```python
from build123d import *

# Parameters (mm, degrees)
ESBO_O1_R                = 3.35
RESSALTO_EXTRUS_O1_DEPTH = 10
ESBO_O2_R                = 1.75
CORTE_EXTRUS_O1_DEPTH    = 10
ESBO_O3_W                = 10.1
ESBO_O3_H                = 5
CORTE_EXTRUS_O2_DEPTH    = 20


with BuildPart() as part:
    # Esboço1 → Ressalto-extrusão1 (new body)
    with BuildSketch(Plane.XY):
        Polygon((-8, -5), (-8, -15), (8, -15), (8, -5), (20, -5), (20, 0), (-20, 0), (-20, -5), align=None)
        with Locations((0, -6.75)):
            Circle(ESBO_O1_R, mode=Mode.SUBTRACT)
    extrude(amount=RESSALTO_EXTRUS_O1_DEPTH)

    # Esboço2 → Corte-extrusão1 (cut)
    with BuildSketch(Plane(origin=(0, 0, 0), x_dir=(1, 0, 0), z_dir=(0, 1, 0))):
        with Locations(Location((-15, -5, 0), (0, 0, 180))):
            Circle(ESBO_O2_R)
        with Locations(Location((15, -5, 0), (0, 0, 180))):
            Circle(ESBO_O2_R)
    extrude(amount=-CORTE_EXTRUS_O1_DEPTH, mode=Mode.SUBTRACT)

    # Esboço3 → Corte-extrusão2 (cut)
    with BuildSketch(Plane.XZ.offset(15)):
        with Locations((0, 5)):
            Rectangle(ESBO_O3_W, ESBO_O3_H)
    extrude(amount=-CORTE_EXTRUS_O2_DEPTH, mode=Mode.SUBTRACT)


solid = part.part
```
Read the model definition and answer for the solid it produces. Units are mm, in the model's axes. A direction names the side the tool comes from. Coordinates: 2 decimals unless noted, no trailing zeros. Write each loop counter-clockwise with the first axis right and the second up, starting at its lowest first coordinate (ties: lowest second). Pieces come first, ordered by that corner, then holes. Notation, with made-up numbers: (30, 16) -> (45, 16) arc R22 ccw to (45, 30) -> close; hole circle Ø3 at (29, 68.5). An arc over 180 degrees is marked (long way). Answer as a JSON object with one key per item and string values.
Q1. The part is cut by section C-C on y = -11.75. Give the vertices of the cut face in (x, z).
The answers:
{"outline": "(-8, 0) -> (8, 0) -> (8, 10) -> (-8, 10) -> close; hole (-5.05, 2.5) -> (5.05, 2.5) -> (5.05, 7.5) -> (-5.05, 7.5) -> close"}
Q2. The part is cut by section A-A on x = -4. Give the vertices of the cut face in (y, z), then the cut area to 3 significant figures.
The answers:
{"outline": "(-15, 0) -> (0, 0) -> (0, 2.5) -> (-15, 2.5) -> close; (-15, 7.5) -> (0, 7.5) -> (0, 10) -> (-15, 10) -> close", "area": "75.0 mm2"}
Q3. Consider line 1 (Y direction, x = 0, z = 1.15); line 2 (X direction, y = -1, z = 5.5); line 3 (Z direction, x = 15, y = -1.85). Determine where each line is inside the solid, lowest interval first. Write a range as [from, to].
The answers:
{"line 1": "y = [-15, -10.1], [-3.4, 0]", "line 2": "x = [-20, -16.68], [-13.32, -5.05], [5.05, 13.32], [16.68, 20]", "line 3": "z = [0, 3.25], [6.75, 10]"}
Q4. Flat-ended cylindrical pins translate along their axes: pin 1 Ø1.5 at (y, z) = (-8.5, 1) entering from +X; pin 2 Ø5 at (y, z) = (-12, 3) entering from -X. Find the tip coordinate at first contact, or state that the pin passes through.
The answers:
{"pin 1": "stops at x = 8", "pin 2": "stops at x = -8"}
Q5. The part is cut by section D-D on z = 3.75. Give the vertices of the cut face in (x, y).
The answers:
{"outline": "(-20, -5) -> (-16.22, -5) -> (-16.22, 0) -> (-20, 0) -> close; (-13.78, -5) -> (-8, -5) -> (-8, -15) -> (-5.05, -15) -> (-5.05, 0) -> (-13.78, 0) -> close; (5.05, -15) -> (8, -15) -> (8, -5) -> (13.78, -5) -> (13.78, 0) -> (5.05, 0) -> close; (16.22, -5) -> (20, -5) -> (20, 0) -> (16.22, 0) -> close"}
Q6. A tool of negligible diameter and unlimited length cuts with its end or side. For faces 1 (the flat face through (13, -5, 5)), 2 (the flat face through (-8, -10, 5)), 3 (the flat face through (5.05, -8, 5)), from which of +Z, -Z, +X, -X, +Y, -Y can it reach the whole face along a straight path? Write none if from no direction.
The answers:
{"face 1": "+Z, -Z, +X, -Y", "face 2": "+Z, -Z, -X, -Y", "face 3": "+Y, -Y"}
Q7. The part is cut by section B-B on x = 0. Give the vertices of the cut face in (y, z).
The answers:
{"outline": "(-15, 0) -> (-10.1, 0) -> (-10.1, 2.5) -> (-15, 2.5) -> close; (-15, 7.5) -> (-10.1, 7.5) -> (-10.1, 10) -> (-15, 10) -> close; (-3.4, 0) -> (0, 0) -> (0, 2.5) -> (-3.4, 2.5) -> close; (-3.4, 7.5) -> (0, 7.5) -> (0, 10) -> (-3.4, 10) -> close"}
Q8. Determine the mould class of faces 4 (the flat face through (0, -11, 7.5)), 5 (the flat face through (0, -2, 10)), 6 (the cylindrical face through (-2.658, -8.788, 8.732)) for opening direction Z: pulls with the +Z half, pulls with the -Z half, needs draft (parallel to the pull), parting line crosses it, or undercut.
The answers:
{"face 4": "undercut", "face 5": "pulls with the +Z half", "face 6": "needs draft"}
